from build123d import *

# Parameters (mm, degrees)
F1_DEPTH    = 38.1
F2_T1_DEPTH = 273.4584537484
F2_T3_DEPTH = 273.4584537484
F3_SIZE     = 12.7
F5_DEPTH    = 6.35
F8_DEPTH    = 12.7
F9_DEPTH    = 38.1


# Not quite as in the source:
# - a fillet or chamfer that OpenCascade refuses, or shapes differently, is made with other operations: its cross-section is extruded or revolved along the edge and cut away or added


with BuildPart() as f1:
    # F0 (on Top) → F1 (new body)
    with BuildSketch(Plane.XY):
        Polygon((0, 63.4811788997), (-44.45, 0), (44.45, 0), align=None)
        Polygon((44.45, 0), (-44.45, 0), (-44.45, -76.2188211003), (-25.4, -76.2188211003), (-25.4, -38.1188211003), (25.4, -38.1188211003), (25.4, -76.2188211003), (44.45, -76.2188211003), align=None)
    extrude(amount=-F1_DEPTH)

    # F2: chamfer of 38.1 on 2 edges, made by hand

    # F2_s2 → F2_t1 (cut)
    with BuildSketch(Plane(origin=(70.8232650101, -101.1461047552, 0), x_dir=(0, 0, 1), z_dir=(-0.5735764364, 0.8191520443, 0))):
        Polygon((0, 36.4113083686), (-38.1, -1.6886916314), (-38.1, 36.4113083686), align=None)
    extrude(amount=F2_T1_DEPTH, mode=Mode.SUBTRACT)

    # F2_s4 → F2_t3 (cut)
    with BuildSketch(Plane(origin=(86.0260603809, 122.8579466609, 0), x_dir=(0, 0, 1), z_dir=(-0.5735764364, -0.8191520443, 0))):
        Polygon((0, 36.4113083686), (-38.1, -1.6886916314), (-38.1, 36.4113083686), align=None)
    extrude(amount=F2_T3_DEPTH, mode=Mode.SUBTRACT)

    # F3
    f3_edges = [f1.edges().sort_by_distance(p)[0] for p in [
        (44.45, -71.322072, -38.1),
        (-44.45, -71.322072, -38.1),
    ]]
    chamfer(f3_edges, length=F3_SIZE)

    # F4 (on Top) → F5 (cut)
    with BuildSketch(Plane.XY):
        with BuildLine():
            ThreePointArc((5.2016154812, 28.8462825899), (0, 31.5540722191), (-5.2016154812, 28.8462825899))
            Line((-5.2016154812, 28.8462825899), (-24.2516154812, 1.6400630614))
            ThreePointArc((-24.2516154812, 1.6400630614), (-25.1061026373, -0.0926654825), (-25.4, -2.0021473094))
            Line((-25.4, -2.0021473094), (-25.4, -25.4188211003))
            ThreePointArc((-25.4, -25.4188211003), (-23.5401280605, -29.9089491608), (-19.05, -31.7688211003))
            Line((-19.05, -31.7688211003), (0, -31.7688211003))
            Line((0, -31.7688211003), (19.05, -31.7688211003))
            ThreePointArc((19.05, -31.7688211003), (23.5401280605, -29.9089491608), (25.4, -25.4188211003))
            Line((25.4, -25.4188211003), (25.4, -2.0021473094))
            ThreePointArc((25.4, -2.0021473094), (25.1061026373, -0.0926654825), (24.2516154812, 1.6400630614))
            Line((24.2516154812, 1.6400630614), (5.2016154812, 28.8462825899))
        make_face()
    extrude(amount=-F5_DEPTH, mode=Mode.SUBTRACT)

    # F7 (on Top) → F8 (cut)
    with BuildSketch(Plane.XY):
        with BuildLine():
            Line((-19.05, -31.7688211003), (0, -31.7688211003))
            Line((0, -31.7688211003), (19.05, -31.7688211003))
            ThreePointArc((19.05, -31.7688211003), (23.5401280605, -29.9089491608), (25.4, -25.4188211003))
            Line((25.4, -25.4188211003), (25.4, -24.1439216138))
            ThreePointArc((25.4, -24.1439216138), (25.1061026373, -22.2344397869), (24.2516154812, -20.5017112429))
            Line((24.2516154812, -20.5017112429), (5.2016154812, 6.7045082855))
            ThreePointArc((5.2016154812, 6.7045082855), (0, 9.4122979147), (-5.2016154812, 6.7045082855))
            Line((-5.2016154812, 6.7045082855), (-24.2516154812, -20.5017112429))
            ThreePointArc((-24.2516154812, -20.5017112429), (-25.1061026373, -22.2344397869), (-25.4, -24.1439216138))
            Line((-25.4, -24.1439216138), (-25.4, -25.4188211003))
            ThreePointArc((-25.4, -25.4188211003), (-23.5401280605, -29.9089491608), (-19.05, -31.7688211003))
        make_face()
    extrude(amount=-F8_DEPTH, mode=Mode.SUBTRACT)

    # F6 (on Right) → F9 (join, symmetric)
    with BuildSketch(Plane.YZ):
        Polygon((-12.7, 12.7), (-12.7, 0), (0, 0), align=None)
    extrude(amount=F9_DEPTH, both=True)


solid = f1.part
Part model, mm, in its own coordinate system. A direction names the side the tool comes from. Coordinates: 2 decimals unless noted, no trailing zeros. Order: outer loops, then holes, each group sorted by start corner. A loop starts at its lowest first (then second) coordinate and runs counter-clockwise, first axis right, second up. Notation, with made-up numbers: M -32.75,40 L -9.75,40 A7 cw -9.75,44 Z; hole C 64,12.25 d1. An arc over 180 degrees is marked long. Use a Markdown table: item, result.
(1) Tool access for faces 4 (the flat face through (14.86, 15.05, -3.13)), 5 (the flat face through (-14.593, -6.708, -9.481)), 6 (the flat face through (24.949, -4.898, -18.783)), 7 (the flat face through (0, -38.119, -19)), 8 (the flat face through (38.1, -9, 4)): list every direction of +Z, -Z, +X, -X, +Y, -Y with a clear straight run to the whole face (end or side of a thin tool).
A:
| item | result |
|---|---|
| face 4 | +Z |
| face 5 | none |
| face 6 | -Z, +X, +Y |
| face 7 | +Z, -Z, -Y |
| face 8 | +Z, +X, +Y, -Y |
(2) Cut at A-A on y = -68. Write the cut outline in (x, z), then the cut area to 3 significant figures.
A:
| item | result |
|---|---|
| outline | M -44.45,-25.4 L -31.75,-38.1 L -25.4,-38.1 L -25.4,0 L -44.45,0 Z; M 25.4,-38.1 L 31.75,-38.1 L 44.45,-25.4 L 44.45,0 L 25.4,0 Z |
| area | 1,290 mm^2 |
(3) Flat gauge pins, fed straight in: pin 1 (2 mm diameter, centred on x = 27, y = 23, fed in from +Z); pin 2 (19 mm diameter, centred on x = -10.5, z = -13.5, fed in from -Y); pin 3 (1 mm diameter, centred on x = -26, y = 26, fed in from -Z). Where does each tip first touch, or does it go through?
A:
| item | result |
|---|---|
| pin 1 | stops at z = 0 |
| pin 2 | stops at y = -38.12 |
| pin 3 | stops at z = -0.7 |
(4) Probe L1, parallel to X at y = -66.5, z = -5; L2, parallel to Z at x = -10, y = -18; L3, parallel to X at y = -47.5, z = -31.5. List the from-to ranges inside material, lowest first.
A:
| item | result |
|---|---|
| L1 | x = -44.45 to -25.4, 25.4 to 44.45 |
| L2 | z = -38.1 to -12.7 |
| L3 | x = -38.35 to -25.4, 25.4 to 38.35 |
(5) Cut at C-C on z = -10. Write the cut outline in (x, y), then the cut area to 3 significant figures.
A:
| item | result |
|---|---|
| outline | M -44.45,-76.22 L -25.4,-76.22 L -25.4,-38.12 L 25.4,-38.12 L 25.4,-76.22 L 44.45,-76.22 L 44.45,-17.43 L 0,46.05 L -44.45,-17.43 Z; hole M -25.4,-25.42 A6.35 ccw -19.05,-31.77 L 19.05,-31.77 A6.35 ccw 25.4,-25.42 L 25.4,-24.14 A6.35 ccw 24.25,-20.5 L 5.2,6.7 A6.35 ccw -5.2,6.7 L -24.25,-20.5 A6.35 ccw -25.4,-24.14 Z |
| area | 4,740 mm^2 |
(6) Cut at B-B on x = 17.5. Write the cut outline in (y, z).
A:
| item | result |
|---|---|
| outline | M -38.12,-38.1 L -27.94,-38.1 L 38.49,0 L 11.28,0 L 11.28,-6.35 L -10.86,-6.35 L -10.86,-12.7 L -31.77,-12.7 L -31.77,0 L -38.12,0 Z; M -12.7,0 L 0,0 L -12.7,12.7 Z |
(7) Cut at D-D on y = 23. Write the cut outline in (x, z).
A:
| item | result |
|---|---|
| outline | M -28.35,0 L 0,-23.22 L 28.35,0 L 9.3,0 L 9.3,-6.35 L -9.3,-6.35 L -9.3,0 Z |
(8) Pull direction Y, two halves, no side cores. Call faces 1 (the flat face through (-24.04, -3.59, -18.78)), 2 (the flat face through (-38.1, -9, 4)), 3 (the flat face through (14.86, -7.09, -9.48)): released by +Y, released by -Y, zero draft, split by the parting line, or undercut.
A:
| item | result |
|---|---|
| face 1 | released by +Y |
| face 2 | zero draft |
| face 3 | undercut |
